from build123d import *

# Parameters (mm, degrees)
BOSS_EXTRUDE1_DEPTH                  = 10
CUT_EXTRUDE1_REACH                   = 76.458
SKETCH2_R                            = 7
CUT_EXTRUDE2_REACH                   = 76.458
SKETCH5_R                            = 4
CHAMFER1_SIZE                        = 0.5
F_4_2_4_2_DIAMETER_HOLE1_D           = 4.2
F_4_2_4_2_DIAMETER_HOLE1_DEPTH       = 8
F_4_2_4_2_DIAMETER_HOLE1_CSINK_D     = 4.25
F_4_2_4_2_DIAMETER_HOLE1_CSINK_ANGLE = 90
F_4_2_4_2_DIAMETER_HOLE1_TIP         = 1.2618073
CUT_EXTRUDE4_REACH                   = 78.446
SKETCH15_R                           = 2.5
SKETCH6_R                            = 1
CUT_EXTRUDE6_DEPTH                   = 21
CUT_EXTRUDE10_DEPTH                  = 2
SKETCH23_R                           = 1.99826656
CUT_EXTRUDE11_DEPTH                  = 30
SKETCH24_R                           = 1
CUT_EXTRUDE12_DEPTH                  = 51
F_3_0_3_DIAMETER_HOLE2_D             = 3
F_3_0_3_DIAMETER_HOLE2_DEPTH         = 8.098709071
F_3_0_3_DIAMETER_HOLE2_CSINK_D       = 3.05
F_3_0_3_DIAMETER_HOLE2_CSINK_ANGLE   = 90
F_3_0_3_DIAMETER_HOLE2_TIP           = 0.901290929
CUT_EXTRUDE13_REACH                  = 76.458
CUT_EXTRUDE13_END_RADIUS             = 7
SKETCH28_R                           = 1.6


with BuildPart() as part:
    # Sketch1 → Boss-Extrude1 (new, symmetric)
    with BuildSketch(Plane.XY):
        Polygon((0, 0), (28, 0), (40, -38), (40, -62), (19, -62), (19, -32), (0, -32), align=None)
    extrude(amount=BOSS_EXTRUDE1_DEPTH, both=True)

    # Sketch2 → Cut-Extrude1 (cut, up to next)
    with BuildSketch(Plane(origin=(0, 0, 0), x_dir=(1, 0, 0), z_dir=(0, 1, 0)), mode=Mode.PRIVATE) as cut_extrude1_sk1:
        with Locations(Location((10, 0, 0), (0, 0, 270))):
            Circle(SKETCH2_R)
    cut_extrude1_tool1 = extrude(cut_extrude1_sk1.sketch, amount=-CUT_EXTRUDE1_REACH, mode=Mode.PRIVATE) & part.part
    add(cut_extrude1_tool1.solids().sort_by_distance((10, 0, 0))[0], mode=Mode.SUBTRACT)

    # Sketch5 → Cut-Extrude2 (cut, up to next)
    with BuildSketch(Plane(origin=(40, 0, 0), x_dir=(0, 0, -1), z_dir=(1, 0, 0)), mode=Mode.PRIVATE) as cut_extrude2_sk1:
        with Locations((0, -52)):
            Circle(SKETCH5_R)
    cut_extrude2_tool1 = extrude(cut_extrude2_sk1.sketch, amount=-CUT_EXTRUDE2_REACH, mode=Mode.PRIVATE) & part.part
    add(cut_extrude2_tool1.solids().sort_by_distance((40, -52, 0))[0], mode=Mode.SUBTRACT)

    # Chamfer1
    chamfer1_edges = [part.edges().sort_by_distance(p)[0] for p in [
        (40, -52, 4),
    ]]
    chamfer(chamfer1_edges, length=CHAMFER1_SIZE)

    # Ø4.2 (4.2) Diameter Hole1
    with Locations(Plane(origin=(0, -62, 0), x_dir=(-1, 0, 0), z_dir=(0, -1, 0))):
        with Locations((-32, 0), (-24, 0)):
            CounterSinkHole(F_4_2_4_2_DIAMETER_HOLE1_D / 2, F_4_2_4_2_DIAMETER_HOLE1_CSINK_D / 2, depth=F_4_2_4_2_DIAMETER_HOLE1_DEPTH, counter_sink_angle=F_4_2_4_2_DIAMETER_HOLE1_CSINK_ANGLE)
            with Locations((0, 0, -(F_4_2_4_2_DIAMETER_HOLE1_DEPTH + F_4_2_4_2_DIAMETER_HOLE1_TIP / 2))):  # 118° drill point
                Cone(0, F_4_2_4_2_DIAMETER_HOLE1_D / 2, F_4_2_4_2_DIAMETER_HOLE1_TIP, mode=Mode.SUBTRACT)

    # Sketch15 → Cut-Extrude4 (cut, up to next)
    with BuildSketch(Plane.XY.offset(10), mode=Mode.PRIVATE) as cut_extrude4_sk1:
        with Locations((32, -42)):
            Circle(SKETCH15_R)
    cut_extrude4_tool1 = extrude(cut_extrude4_sk1.sketch, amount=-CUT_EXTRUDE4_REACH, mode=Mode.PRIVATE) & part.part
    add(cut_extrude4_tool1.solids().sort_by_distance((32, -42, 10))[0], mode=Mode.SUBTRACT)

    # Sketch6 → Cut-Extrude6 (cut)
    with BuildSketch(Plane.XZ.offset(62)):
        with Locations(Location((32, 0, 0), (0, 0, 270))):
            Circle(SKETCH6_R)
    extrude(amount=-CUT_EXTRUDE6_DEPTH, mode=Mode.SUBTRACT)

    # Sketch22 → Cut-Extrude10 (cut)
    with BuildSketch(Plane(origin=(0, 0, 0), x_dir=(1, 0, 0), z_dir=(0, 1, 0))):
        with BuildLine():
            ThreePointArc((16.708203932, 2), (17, 0), (16.708203932, -2))
            Line((16.708203932, -2), (24, -2))
            ThreePointArc((24, -2), (26, 0), (24, 2))
            Line((24, 2), (16.708203932, 2))
        make_face()
    extrude(amount=-CUT_EXTRUDE10_DEPTH, mode=Mode.SUBTRACT)

    # Sketch23 → Cut-Extrude11 (cut)
    with BuildSketch(Plane(origin=(0, 0, 0), x_dir=(1, 0, 0), z_dir=(0, 1, 0))):
        with Locations(Location((24, 0, 0), (0, 0, 270))):
            Circle(SKETCH23_R)
    extrude(amount=-CUT_EXTRUDE11_DEPTH, mode=Mode.SUBTRACT)

    # Sketch24 → Cut-Extrude12 (cut)
    with BuildSketch(Plane(origin=(0, 0, 0), x_dir=(1, 0, 0), z_dir=(0, 1, 0))):
        with Locations(Location((24, 0, 0), (0, 0, 270))):
            Circle(SKETCH24_R)
    extrude(amount=-CUT_EXTRUDE12_DEPTH, mode=Mode.SUBTRACT)

    # Ø3.0 (3) Diameter Hole2
    with Locations(Plane(origin=(0, 0, 0), x_dir=(1, 0, 0), z_dir=(0, 1, 0))):
        with Locations((24, 7), (24, -6.880303923), (3, -7), (3, 7)):
            CounterSinkHole(F_3_0_3_DIAMETER_HOLE2_D / 2, F_3_0_3_DIAMETER_HOLE2_CSINK_D / 2, depth=F_3_0_3_DIAMETER_HOLE2_DEPTH, counter_sink_angle=F_3_0_3_DIAMETER_HOLE2_CSINK_ANGLE)
            with Locations((0, 0, -(F_3_0_3_DIAMETER_HOLE2_DEPTH + F_3_0_3_DIAMETER_HOLE2_TIP / 2))):  # 118° drill point
                Cone(0, F_3_0_3_DIAMETER_HOLE2_D / 2, F_3_0_3_DIAMETER_HOLE2_TIP, mode=Mode.SUBTRACT)

    # Cut-Extrude13: up to this cylinder (the profile starts outside it)
    cut_extrude13_end = Plane(origin=(10, -17.1005185, 0), z_dir=(0, 1, 0)) * Cylinder(CUT_EXTRUDE13_END_RADIUS, 168.117037, mode=Mode.PRIVATE)
    # Sketch28 → Cut-Extrude13 (cut, up to the surface)
    with BuildSketch(Plane.ZY, mode=Mode.PRIVATE) as cut_extrude13_sk1:
        with Locations((-3, -17)):
            Circle(SKETCH28_R)
    cut_extrude13_tool1 = extrude(cut_extrude13_sk1.sketch, amount=-CUT_EXTRUDE13_REACH, mode=Mode.PRIVATE) - cut_extrude13_end
    add(cut_extrude13_tool1.solids().sort_by_distance((0, -17, -3))[0], mode=Mode.SUBTRACT)
    # Sketch28 → Cut-Extrude13 (cut, up to the surface)
    with BuildSketch(Plane.ZY, mode=Mode.PRIVATE) as cut_extrude13_sk2:
        with Locations((3, -17.201037224)):
            Circle(SKETCH28_R)
    cut_extrude13_tool2 = extrude(cut_extrude13_sk2.sketch, amount=-CUT_EXTRUDE13_REACH, mode=Mode.PRIVATE) - cut_extrude13_end
    add(cut_extrude13_tool2.solids().sort_by_distance((0, -17.201037, 3))[0], mode=Mode.SUBTRACT)


solid = part.part
The model under review builds one solid part; all positions refer to its coordinate system, in mm. A direction names the side the tool comes from. Coordinates: 2 decimals unless noted, no trailing zeros. Loops run counter-clockwise (first coordinate to the right, second up) from the corner with the lowest first, then second, coordinate; pieces in that order, holes last. Notation, with made-up numbers: M 13,-10 L 21,-10 A23 cw 21,23 Z; hole C -16.5,85 d2. An arc over 180 degrees is marked long. Put each result on its own line as item: value. Start each with the question number.
Q1. Add section D-D (y = -29). Write out the cut boundary in (x, z), and give its area (3 significant figures).
Q2. Add section A-A (y = -36.5). Write out the cut boundary in (x, z), and give its area (3 significant figures).
Q3. Wall thickness on line 1 (Z direction, x = 1, y = -17); line 2 (Z direction, x = 32, y = -46.7); line 3 (Z direction, x = 32, y = -59.75): over which ranges is each line inside the solid? List them lowest first.
Q4. Add section B-B (x = 36.5). Write out the cut boundary in (y, z), and give its area (3 significant figures).
Q5. Clearance check with flat-ended pins moving along their axes: pin 1 (5 mm diameter, centred on y = -17, z = -3, fed in from +X); pin 2 (2.5 mm diameter, centred on x = 24, z = 0, fed in from -Y); pin 3 (10 mm diameter, centred on x = 11.5, z = -7, fed in from -Y). State where each tip first meets the part, or that it passes through.
Q6. For faces 1 (the cylindrical face through (29.394, -48.034, 0.521)), 2 (the cylindrical face through (25.5, -4.12, 6.81)), list the 3-axis set-ups (+Z, -Z, +X, -X, +Y, -Y) from which the entire face can be reached by the end or side of a thin tool; tool diameter is ignored.
Q7. The part is to be moulded in two halves that separate along X. For faces 3 (the cylindrical face through (33.94, -58.64, 0.8)), 4 (the flat face through (34, -19, 0)), 5 (the flat face through (20, -31, 10)), 6 (the flat face through (20, -1, 2)), say which applies: +X half, -X half, draft (parallel to the pull), parting line (faces both ways), or undercut.
Q8. Add section C-C (z = 0). Count the separate pieces of the cut face and the enclosed holes in it, and give its area (3 significant figures).
Answers:
1. outline: M 0,-10 L 37.16,-10 L 37.16,10 L 0,10 Z; hole C 10,0 d14; hole C 24,0 d4
1. area: 577 mm^2
2. outline: M 19,-10 L 39.53,-10 L 39.53,10 L 19,10 Z; hole C 24,0 d2
2. area: 407 mm^2
3. line 1: z = -10 to -4.6, -1.4 to 1.41, 4.59 to 10
3. line 2: z = -10 to -1, 1 to 10
3. line 3: z = -10 to -2.1, 2.1 to 10
4. outline: M -62,-10 L -26.92,-10 L -26.92,10 L -62,10 Z; hole C -52,0 d8
4. area: 651 mm^2
5. pin 1: stops at x = 34.16
5. pin 2: stops at y = -48.2
5. pin 3: stops at y = -32
6. face 1: +X, -X
6. face 2: +Y
7. face 3: undercut
7. face 4: +X half
7. face 5: draft
7. face 6: undercut
8. separate pieces: 6
8. enclosed holes: 0
8. area: 823 mm^2
